from build123d import *

# Parameters (mm, degrees)
BOSS_EXTRUDE1_DEPTH = 6.35
CUT_EXTRUDE1_REACH  = 8.35
SKETCH2_W           = 29.21
SKETCH2_H           = 29.21
FILLET1_R           = 5.08
BOSS_EXTRUDE2_DEPTH = 6.35
FILLET2_R           = 5.08


with BuildPart() as part:
    # Sketch1 → Boss-Extrude1 (new body)
    with BuildSketch(Plane.XY):
        with BuildLine():
            ThreePointArc((-68.188405154, 82.55), (-87.437503618, 43.287282526), (-95.244575115, 0.262424481))
            ThreePointArc((-95.244575115, 0.262424481), (0, -99.003097439), (95.244575115, 0.262424481))
            ThreePointArc((95.244575115, 0.262424481), (87.437503618, 43.287282526), (68.188405154, 82.55))
            ThreePointArc((68.188405154, 82.55), (0, 118.781058361), (-68.188405154, 82.55))
        make_face()
        with BuildLine():
            Line((-64.77, 76.2), (64.77, 76.2))
            ThreePointArc((64.77, 76.2), (81.91955238, 39.710108254), (88.9, 0))
            ThreePointArc((88.9, 0), (0, -92.653098722), (-88.9, 0))
            ThreePointArc((-88.9, 0), (-81.91955238, 39.710108254), (-64.77, 76.2))
        make_face(mode=Mode.SUBTRACT)
    extrude(amount=BOSS_EXTRUDE1_DEPTH)

    # Sketch2 → Cut-Extrude1 (cut, up to next)
    with BuildSketch(Plane.XY.offset(6.35), mode=Mode.PRIVATE) as cut_extrude1_sk1:
        with Locations((0, 97.49052918)):
            Rectangle(SKETCH2_W, SKETCH2_H)
    cut_extrude1_tool1 = extrude(cut_extrude1_sk1.sketch, amount=-CUT_EXTRUDE1_REACH, mode=Mode.PRIVATE) & part.part
    add(cut_extrude1_tool1.solids().sort_by_distance((0, 97.490529, 6.35))[0], mode=Mode.SUBTRACT)

    # Fillet1
    fillet1_edges = [part.edges().sort_by_distance(p)[0] for p in [
        (14.605, 112.09552918, 3.175),
        (14.605, 82.88552918, 3.175),
        (-14.605, 82.88552918, 3.175),
        (-14.605, 112.09552918, 3.175),
    ]]
    fillet(fillet1_edges, radius=FILLET1_R)

    # Sketch3 → Boss-Extrude2 (add)
    with BuildSketch(Plane.XY.offset(6.35)):
        with BuildLine():
            ThreePointArc((-64.77, 76.2), (-65.301178837, 75.369054935), (-65.826969345, 74.534689907))
            Line((-65.826969345, 74.534689907), (0.397744119, 2.447786681))
            Line((0.397744119, 2.447786681), (2.867484972, 5.391109215))
            Line((2.867484972, 5.391109215), (-62.183145491, 76.2))
            Line((-62.183145491, 76.2), (-64.77, 76.2))
        make_face()
        with BuildLine():
            Line((62.283199114, 76.2), (2.867484972, 5.391109215))
            Line((2.867484972, 5.391109215), (5.466869825, 2.561627672))
            Line((5.466869825, 2.561627672), (65.84083728, 74.512520285))
            ThreePointArc((65.84083728, 74.512520285), (65.308184865, 75.358015528), (64.77, 76.2))
            Line((64.77, 76.2), (62.283199114, 76.2))
        make_face()
        with BuildLine():
            Line((5.466869825, 2.561627672), (2.997128973, -0.381694862))
            Line((2.997128973, -0.381694862), (63.387167907, -66.117440095))
            ThreePointArc((63.387167907, -66.117440095), (64.712838285, -64.7424562), (66.008689372, -63.339333743))
            Line((66.008689372, -63.339333743), (5.466869825, 2.561627672))
        make_face()
        Polygon((2.867484972, 5.391109215), (0.397744119, 2.447786681), (2.997128973, -0.381694862), (5.466869825, 2.561627672), align=None)
        with BuildLine():
            Line((2.997128973, -0.381694862), (0.397744119, 2.447786681))
            Line((0.397744119, 2.447786681), (-59.927506787, -69.445047811))
            ThreePointArc((-59.927506787, -69.445047811), (-58.505389643, -70.713272134), (-57.056440469, -71.950751993))
            Line((-57.056440469, -71.950751993), (2.997128973, -0.381694862))
        make_face()
    extrude(amount=-BOSS_EXTRUDE2_DEPTH)

    # Fillet2
    fillet2_edges = [part.edges().sort_by_distance(p)[0] for p in [
        (0.397744119, 2.447786681, 3.175),
        (-65.826969345, 74.534689907, 3.175),
        (-62.183145491, 76.2, 3.175),
        (2.867484972, 5.391109215, 3.175),
        (62.283199114, 76.2, 3.175),
        (65.84083728, 74.512520285, 3.175),
        (5.466869825, 2.561627672, 3.175),
        (66.008689372, -63.339333743, 3.175),
        (63.387167907, -66.117440095, 3.175),
        (2.997128973, -0.381694862, 3.175),
        (-57.056440469, -71.950751993, 3.175),
        (-59.927506787, -69.445047811, 3.175),
    ]]
    fillet(fillet2_edges, radius=FILLET2_R)


solid = part.part
Geometry check sheet. Reference: the model listing, model coordinates, mm. A direction names the side the tool comes from. Give positions to 0.01 mm unless a question says otherwise; leave off trailing zeros. Order: outer loops, then holes, each group sorted by start corner. A loop starts at its lowest first (then second) coordinate and runs counter-clockwise, first axis right, second up.
1) Draft check along Y on faces 3 (the cylindrical face through (1.125, 118.773, 3.131)), 4 (the flat face through (28, 35, 0)), 5 (the flat face through (0, 82.886, 3)). Enter one of: released by +Y, released by -Y, zero draft, split by the parting line, or undercut.
Results are:
face 3: released by +Y
face 4: zero draft
face 5: undercut
2) Cross-section at D-D (x = -6.5). Record the boundary of the cut face in (y, z).
Results are:
outline: (-98.78, 0) - (-92.42, 0) - (-92.42, 6.35) - (-98.78, 6.35) - close; (-11.7, 0) - (-5.77, 0) - (-5.77, 6.35) - (-11.7, 6.35) - close; (9.96, 0) - (15.59, 0) - (15.59, 6.35) - (9.96, 6.35) - close; (76.2, 0) - (82.89, 0) - (82.89, 6.35) - (76.2, 6.35) - close; (112.1, 0) - (118.52, 0) - (118.52, 6.35) - (112.1, 6.35) - close
3) Cross-section at B-B (y = 60). Record the boundary of the cut face in (x, z), then the cut area to 3 significant figures.
Results are:
outline: (-80.87, 0) - (-73.85, 0) - (-73.85, 6.35) - (-80.87, 6.35) - close; (-52.47, 0) - (-47.3, 0) - (-47.3, 6.35) - (-52.47, 6.35) - close; (48.69, 0) - (53.66, 0) - (53.66, 6.35) - (48.69, 6.35) - close; (73.85, 0) - (80.87, 0) - (80.87, 6.35) - (73.85, 6.35) - close
area: 154 mm2
4) Gauge pin test, flat ends, axial feed: pin 1 (1.9 mm diameter, centred on x = 4.5, z = 2, fed in from -Y); pin 2 (1.5 mm diameter, centred on y = -56.5, z = 1.5, fed in from -X); pin 3 (1.5 mm diameter, centred on x = 47, z = 1.5, fed in from -Y). Record the tip position at first contact, or that the pin passes through.
Results are:
pin 1: stops at y = -98.94
pin 2: stops at x = -79.85
pin 3: stops at y = -87.03
5) Tool access check on faces 1 (the cylindrical face through (-87.245, 43.87, 3.131)), 2 (the cylindrical face through (-54.845, -71.742, 3.131)). Record the directions out of +Z, -Z, +X, -X, +Y, -Y that give a thin tool (end or side, any length) a straight path to the whole face; none if there is none.
Results are:
face 1: +Z, -Z, -X, +Y
face 2: +Z, -Z
6) Material ranges on probe 1 along X at (y, z) = (67, 3.75) (3 decimals); probe 2 along X at (y, z) = (12.5, 4.75); probe 3 along Y at (x, z) = (-34, 0.5), recorded low to high.
Results are:
probe 1: x = -77.445 to -70.246, -58.905 to -53.731, 54.563 to 59.537, 70.246 to 77.445
probe 2: x = -94.26 to -87.87, -8.84 to -3.66, 8.83 to 13.81, 87.87 to 94.26
probe 3: y = -92.73 to -85.9, -44.47 to -38.55, 39.89 to 45.52, 76.2 to 111.43
7) Cross-section at A-A (x = -77). Record the boundary of the cut face in (y, z), then the cut area to 3 significant figures.
Results are:
outline: (-59.87, 0) - (-48.26, 0) - (-48.26, 6.35) - (-59.87, 6.35) - close; (53.05, 0) - (67.85, 0) - (67.85, 6.35) - (53.05, 6.35) - close
area: 168 mm2
8) Cross-section at C-C (x = 33.5). Record the boundary of the cut face in (y, z).
Results are:
outline: (-92.92, 0) - (-86.11, 0) - (-86.11, 6.35) - (-92.92, 6.35) - close; (-33.58, 0) - (-27.95, 0) - (-27.95, 6.35) - (-33.58, 6.35) - close; (35.97, 0) - (41.9, 0) - (41.9, 6.35) - (35.97, 6.35) - close; (76.2, 0) - (111.65, 0) - (111.65, 6.35) - (76.2, 6.35) - close
